from build123d import *

# Parameters (mm, degrees)
PAD_DEPTH = 10
FILLET_R  = 0.8


with BuildPart() as part:
    # Sketch → Pad (new body)
    with BuildSketch(Plane.XY):
        Polygon((-1, 0), (-1.8, 100), (1.8, 100), (1, 0), align=None)
    extrude(amount=PAD_DEPTH)

    # Fillet
    fillet_edges = [part.edges().sort_by_distance(p)[0] for p in [
        (-1.8, 100, 5),
        (1.8, 100, 5),
        (-1, 0, 5),
        (1, 0, 5),
    ]]
    fillet(fillet_edges, radius=FILLET_R)


solid = part.part
Source: CAD feature listing. Evaluate the final solid. Frame: model axes, mm. Coordinates: 2 decimals unless noted, no trailing zeros. Order: outer loops, then holes, each group sorted by start corner. A loop starts at its lowest first (then second) coordinate and runs counter-clockwise, first axis right, second up.
Item 1: Cut plane A-A (z = 7). Return loops of the section in (x, y), plus the area to 3 significant figures.
Output values:
outline: (-1.79, 99.19) - (-1.01, 0.79) arc R0.8 ccw to (-0.21, 0) - (0.21, 0) arc R0.8 ccw to (1.01, 0.79) - (1.79, 99.19) arc R0.8 ccw to (0.99, 100) - (-0.99, 100) arc R0.8 ccw to start
area: 279 mm2
Item 2: Cut plane B-B (y = 62.5). Return loops of the section in (x, z).
Output values:
outline: (-1.5, 0) - (1.5, 0) - (1.5, 10) - (-1.5, 10) - close
Item 3: Cut plane C-C (y = 14). Return loops of the section in (x, z), plus the area to 3 significant figures.
Output values:
outline: (-1.11, 0) - (1.11, 0) - (1.11, 10) - (-1.11, 10) - close
area: 22.2 mm2
Item 4: Material intervals for line 1 (Y direction, x = -0.35, z = 9); line 2 (Y direction, x = 0.9, z = 0.5); line 3 (X direction, y = 11.5, z = 4), sorted ascending.
Output values:
line 1: y = 0.01 to 100
line 2: y = 0.4 to 100
line 3: x = -1.09 to 1.09
Item 5: First-contact query: P1, Ø5, axis at y = 40, z = 3.5, coming from the -X side; P2, Ø4, axis at y = 80.5, z = 6.5, coming from the -X side; P3, Ø1.5, axis at y = 72.5, z = 7, coming from the -X side. Flat tips, straight axial feed; report the tip coordinate or a pass-through.
Output values:
P1: stops at x = -1.34
P2: stops at x = -1.66
P3: stops at x = -1.59
